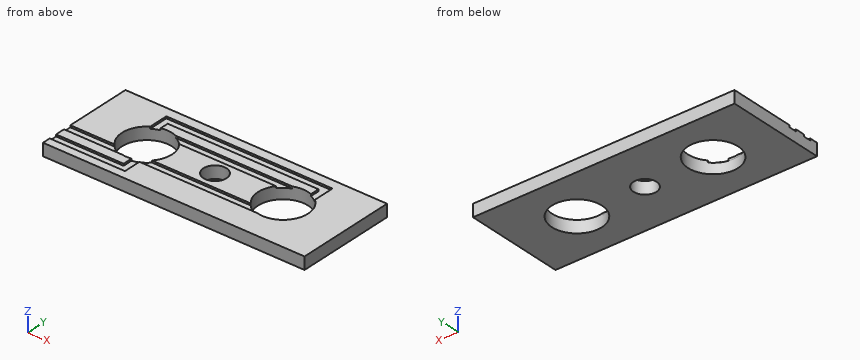
from build123d import *

# Parameters (mm, degrees)
F0_W     = 34
F0_H     = 13
F1_DEPTH = 1.6
F2_R     = 3.25
F3_DEPTH = 1.601
F4_R     = 1.5
F5_DEPTH = 1.601
F7_DEPTH = 0.25


with BuildPart() as f1:
    # F0 (on Top) → F1 (new body)
    with BuildSketch(Plane.XY):
        Rectangle(F0_W, F0_H)
    extrude(amount=F1_DEPTH)

    # F2 (on face) → F3 (cut, through all)
    with BuildSketch(Plane.XY.offset(1.6)):
        with Locations((-8.85, 0)):
            Circle(F2_R)
        with Locations((8.85, 0)):
            Circle(F2_R)
    extrude(amount=-F3_DEPTH, mode=Mode.SUBTRACT)

    # F4 (on face) → F5 (cut, through all)
    with BuildSketch(Plane.XY.offset(1.6)):
        Circle(F4_R)
    extrude(amount=-F5_DEPTH, mode=Mode.SUBTRACT)

    # F6 (on face) → F7 (cut)
    with BuildSketch(Plane.XY.offset(1.6)):
        with BuildLine():
            ThreePointArc((-10.6551859497, 2.7025550294), (-10.1741098428, 2.9680352296), (-9.6551859497, 3.1486783873))
            Line((-9.6551859497, 3.1486783873), (-9.6551859497, 4.25))
            Line((-9.6551859497, 4.25), (9.9456183744, 4.25))
            Line((9.9456183744, 4.25), (9.9456183744, 3.0597582221))
            ThreePointArc((9.9456183744, 3.0597582221), (10.4713685624, 2.8166760525), (10.9456183744, 2.4841263311))
            Line((10.9456183744, 2.4841263311), (10.9456183744, 5.25))
            Line((10.9456183744, 5.25), (-10.6551859497, 5.25))
            Line((-10.6551859497, 5.25), (-10.6551859497, 2.7025550294))
        make_face()
        with BuildLine():
            ThreePointArc((-8.4051859497, 3.2194161677), (-9.0336244397, 3.244808479), (-9.6551859497, 3.1486783873))
            ThreePointArc((-9.6551859497, 3.1486783873), (-10.1741098428, 2.9680352296), (-10.6551859497, 2.7025550294))
            ThreePointArc((-10.6551859497, 2.7025550294), (-12.0760849491, 0.3935427562), (-11.2519368041, -2.1893377055))
            ThreePointArc((-11.2519368041, -2.1893377055), (-10.4439217685, -2.8322982534), (-9.475, -3.1893377055))
            ThreePointArc((-9.475, -3.1893377055), (-8.85, -3.25), (-8.225, -3.1893377055))
            ThreePointArc((-8.225, -3.1893377055), (-7.7095021463, -3.0433147464), (-7.225, -2.8145825623))
            ThreePointArc((-7.225, -2.8145825623), (-6.7923319785, -2.5156514689), (-6.4135405563, -2.1508522448))
            ThreePointArc((-6.4135405563, -2.1508522448), (-5.8101814863, -1.1497840684), (-5.6, 0))
            ThreePointArc((-5.6, 0), (-5.7768788262, 1.0575567367), (-6.2882623085, 2))
            ThreePointArc((-6.2882623085, 2), (-6.8796355522, 2.5846013122), (-7.6, 3))
            Line((-7.6, 3), (-8.4051859497, 3))
            Line((-8.4051859497, 3), (-8.4051859497, 3.2194161677))
        make_face()
        with BuildLine():
            Line((7.6, 3), (-7.6, 3))
            ThreePointArc((-7.6, 3), (-6.8796355522, 2.5846013122), (-6.2882623085, 2))
            Line((-6.2882623085, 2), (6.2882623085, 2))
            ThreePointArc((6.2882623085, 2), (6.8796355522, 2.5846013122), (7.6, 3))
        make_face()
        with BuildLine():
            ThreePointArc((8.0533632375, -3.1508522448), (7.1578925065, -2.774756247), (6.4135405563, -2.1508522448))
            Line((6.4135405563, -2.1508522448), (-6.4135405563, -2.1508522448))
            ThreePointArc((-6.4135405563, -2.1508522448), (-6.7923319785, -2.5156514689), (-7.225, -2.8145825623))
            Line((-7.225, -2.8145825623), (-7.225, -3.1508522448))
            Line((-7.225, -3.1508522448), (8.0533632375, -3.1508522448))
        make_face()
        with BuildLine():
            ThreePointArc((-7.225, -2.8145825623), (-7.7095021463, -3.0433147464), (-8.225, -3.1893377055))
            Line((-8.225, -3.1893377055), (-8.225, -4.4393377055))
            Line((-8.225, -4.4393377055), (-17, -4.4393377055))
            Line((-17, -4.4393377055), (-17, -5.4393377055))
            Line((-17, -5.4393377055), (-7.225, -5.4393377055))
            Line((-7.225, -5.4393377055), (-7.225, -3.1508522448))
            Line((-7.225, -3.1508522448), (-7.225, -2.8145825623))
        make_face()
        with BuildLine():
            ThreePointArc((-9.475, -3.1893377055), (-10.4439217685, -2.8322982534), (-11.2519368041, -2.1893377055))
            Line((-11.2519368041, -2.1893377055), (-17, -2.1893377055))
            Line((-17, -2.1893377055), (-17, -3.1893377055))
            Line((-17, -3.1893377055), (-9.475, -3.1893377055))
        make_face()
    extrude(amount=-F7_DEPTH, mode=Mode.SUBTRACT)


solid = f1.part
Source: CAD feature listing. Evaluate the final solid. Frame: model axes, mm. Round coordinates to 2 decimals unless told otherwise and drop trailing zeros. Order: outer loops, then holes, each group sorted by start corner. A loop starts at its lowest first (then second) coordinate and runs counter-clockwise, first axis right, second up. Notation, with made-up numbers: (-34.5, 83) - (1.5, 83) arc R11 ccw to (1.5, 97) - close; hole circle Ø9 at (-7, 74.5). An arc over 180 degrees is marked (long way). Use a Markdown table: item, result. Add a question column.
1. Section query D-D (x = -8.85). Return the cut outline in (y, z), then the cut area to 3 significant figures.
2. Section query C-C (z = 0.85). Return the cut outline in (x, y), then the cut area to 3 significant figures.
3. Section query A-A (y = 0). Return the cut outline in (x, z), then the cut area to 3 significant figures.
4. Section query B-B (x = 0). Return the cut outline in (y, z).
5. Line query: probe 1 along Y at (x, z) = (-8.85, 0.95); probe 2 along Y at (x, z) = (0, 0.8); probe 3 along X at (y, z) = (-1, 1.4). Output: solid intervals per line, ascending.
6. First-contact query: pin 1 (0.5 mm diameter, centred on x = -14, y = -2.5, fed in from +Z). Flat tip, straight axial feed; report the tip coordinate or a pass-through.
Derived:
| question | item | result |
|---|---|---|
| 1 | outline | (-6.5, 0) - (-3.25, 0) - (-3.25, 1.6) - (-4.44, 1.6) - (-4.44, 1.35) - (-5.44, 1.35) - (-5.44, 1.6) - (-6.5, 1.6) - close; (3.25, 0) - (6.5, 0) - (6.5, 1.6) - (5.25, 1.6) - (5.25, 1.35) - (4.25, 1.35) - (4.25, 1.6) - (3.25, 1.6) - close |
| 1 | area | 9.90 mm2 |
| 2 | outline | (-17, -6.5) - (17, -6.5) - (17, 6.5) - (-17, 6.5) - close; hole circle Ø6.5 at (-8.85, 0); hole circle Ø3 at (0, 0); hole circle Ø6.5 at (8.85, 0) |
| 2 | area | 369 mm2 |
| 3 | outline | (-17, 0) - (-12.1, 0) - (-12.1, 1.6) - (-17, 1.6) - close; (-5.6, 0) - (-1.5, 0) - (-1.5, 1.6) - (-5.6, 1.6) - close; (1.5, 0) - (5.6, 0) - (5.6, 1.6) - (1.5, 1.6) - close; (12.1, 0) - (17, 0) - (17, 1.6) - (12.1, 1.6) - close |
| 3 | area | 28.8 mm2 |
| 4 | outline | (-6.5, 0) - (-1.5, 0) - (-1.5, 1.6) - (-2.15, 1.6) - (-2.15, 1.35) - (-3.15, 1.35) - (-3.15, 1.6) - (-6.5, 1.6) - close; (1.5, 0) - (6.5, 0) - (6.5, 1.6) - (5.25, 1.6) - (5.25, 1.35) - (4.25, 1.35) - (4.25, 1.6) - (3, 1.6) - (3, 1.35) - (2, 1.35) - (2, 1.6) - (1.5, 1.6) - close |
| 5 | probe 1 | -6.5 to -3.25, 3.25 to 6.5 |
| 5 | probe 2 | -6.5 to -1.5, 1.5 to 6.5 |
| 5 | probe 3 | -17 to -11.94, -5.76 to -1.12, 1.12 to 5.76, 11.94 to 17 |
| 6 | pin 1 | z = 1.35 |
